Solid Edge part; units mm, degrees
sketch "Sketch1" plane through (0, 0, 0) normal (0, 0, 1) x (1, 0, 0)
  line L0 (-37.5, -26) -> (37.5, -26)
  line L1 (37.5, -26) -> (37.5, 26)
  line L2 (37.5, 26) -> (-37.5, 26)
  line L3 (-37.5, 26) -> (-37.5, -26)
  circle A0 centre (27.5, -16) radius 5
  circle A1 centre (27.5, 16) radius 5
  circle A2 centre (-27.5, -16) radius 5
  circle A3 centre (-27.5, 16) radius 5
extrude "Protrusion1" add sketch "Sketch1" along normal blind 15
sketch "Sketch2" plane through (0, 0, 0) normal (0, -1, 0) x (1, 0, 0)
  line L0 (-12.5, 15) -> (-12.5, 25)
  arc A0 (-12.5, 25) -> (-2.5, 35) centre (-2.5, 25) cw
  line L1 (7.497, 35) -> (-2.5, 35)
  line L2 (7.497, 55) -> (7.497, 35)
  line L3 (-2.5, 55) -> (7.497, 55)
  arc A1 (-32.5, 25) -> (-2.5, 55) centre (-2.5, 25) cw
  line L4 (-32.5, 15) -> (-32.5, 25)
extrude "ExtrudedProtrusion_2" add sketch "Sketch2" along normal mid plane 12 material side at (-12.55, 0, 20)
sketch "Sketch3" plane through (2.4985, 0, 55) normal (0, 0, 1) x (1, 0, 0)
  circle A0 centre (20.0015, 0) radius 16
  circle A1 centre (20.0015, 0) radius 8
extrude "ExtrudedProtrusion_3" add sketch "Sketch3" against normal blind 20
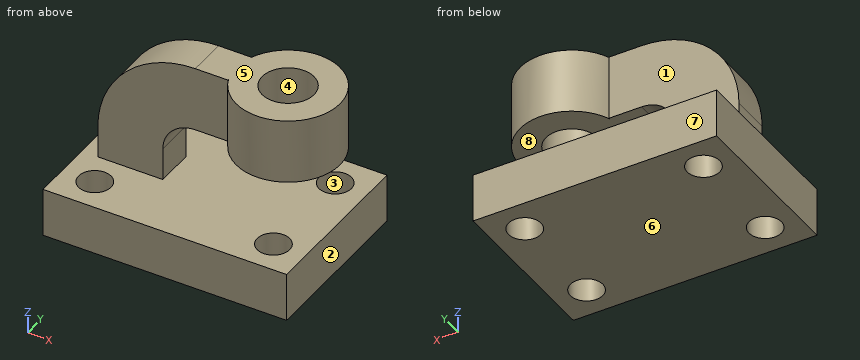
Source: CAD feature listing. Evaluate the final solid. Frame: model axes, mm. Face numbers are marked on the shaded views. A direction names the side the tool comes from. Round coordinates to 2 decimals unless told otherwise and drop trailing zeros. Loops run counter-clockwise (first coordinate to the right, second up) from the corner with the lowest first, then second, coordinate; pieces in that order, holes last. Notation, with made-up numbers: (46.5, 88) - (93.5, 88) arc R19 cw to (93.5, 105) - close; hole circle Ø8 at (61, 72). An arc over 180 degrees is marked (long way). Use CSV: the item, a comma, the result in double quotes.
Q1. Section query A-A, the plane z = 10.5. Output: boundary loops of the cut face in (x, y).
Reported:
outline,"(-37.5, -26) - (37.5, -26) - (37.5, 26) - (-37.5, 26) - close; hole circle Ø10 at (-27.5, -16); hole circle Ø10 at (-27.5, 16); hole circle Ø10 at (27.5, -16); hole circle Ø10 at (27.5, 16)"
Q2. Section query B-B, the plane x = 4.5. Output: boundary loops of the cut face in (y, z), then the cut area to 3 significant figures.
Reported:
outline,"(-26, 0) - (26, 0) - (26, 15) - (-26, 15) - close; (-6, 35) - (6, 35) - (6, 55) - (-6, 55) - close"
area,"1,020 mm^2"
Q3. Ray query, line 1 along Y through (x, z) = (-27.5, 5.5); line 2 along Z through (x, y) = (-3, 4); line 3 along X through (y, z) = (-17.5, 8.5). Return the intervals inside material, ascending.
Reported:
line 1,"-26 to -21, -11 to 11, 21 to 26"
line 2,"0 to 15, 34.99 to 55"
line 3,"-37.5 to -32.27, -22.73 to 22.73, 32.27 to 37.5"
Q4. Mould query, pull axis Z, two halves, no side actions, for the marked faces 5, 6, 7 and 8. Classes: pulls with the +Z half, pulls with the -Z half, needs draft (parallel to the pull), parting line crosses it, or undercut.
Reported:
face 5,"pulls with the +Z half"
face 6,"pulls with the -Z half"
face 7,"needs draft"
face 8,"undercut"
Q5. Section query C-C, the plane y = 0. Output: boundary loops of the cut face in (x, z).
Reported:
outline,"(-37.5, 0) - (37.5, 0) - (37.5, 15) - (-12.5, 15) - (-12.5, 25) arc R10 cw to (-2.5, 35) - (14.5, 35) - (14.5, 55) - (-2.5, 55) arc R30 ccw to (-32.5, 25) - (-32.5, 15) - (-37.5, 15) - close; (30.5, 35) - (38.5, 35) - (38.5, 55) - (30.5, 55) - close"
Q6. Pin query (flat end, axial travel): pin 1 Ø5 at (y, z) = (12.5, 43.5) entering from +X; pin 2 Ø11 at (y, z) = (0.5, 22) entering from -X; pin 3 Ø5 at (y, z) = (-9.5, 33) entering from -X. Return the tip coordinate at first contact, or that it passes through.
Reported:
pin 1,"x = 34.99"
pin 2,"x = -32.5"
pin 3,"x = 8.64"
Q7. Section query D-D, the plane z = 43. Output: boundary loops of the cut face in (x, y), then the cut area to 3 significant figures.
Reported:
outline,"(-26.5, -6) - (7.5, -6) - (7.5, -5.56) arc R16 ccw (long way) to (7.5, 5.56) - (7.5, 6) - (-26.5, 6) - close; hole circle Ø16 at (22.5, 0)"
area,"1,000 mm^2"
Q8. Reachability of the marked faces 1, 2, 3 and 4 from +Z, -Z, +X, -X, +Y, -Y: full face, straight path, thin tool, end or side. Return the list, or none.
Reported:
face 1,"+Z, -X, +Y"
face 2,"-Z, +X, +Y, -Y"
face 3,"-Z"
face 4,"+Z"
